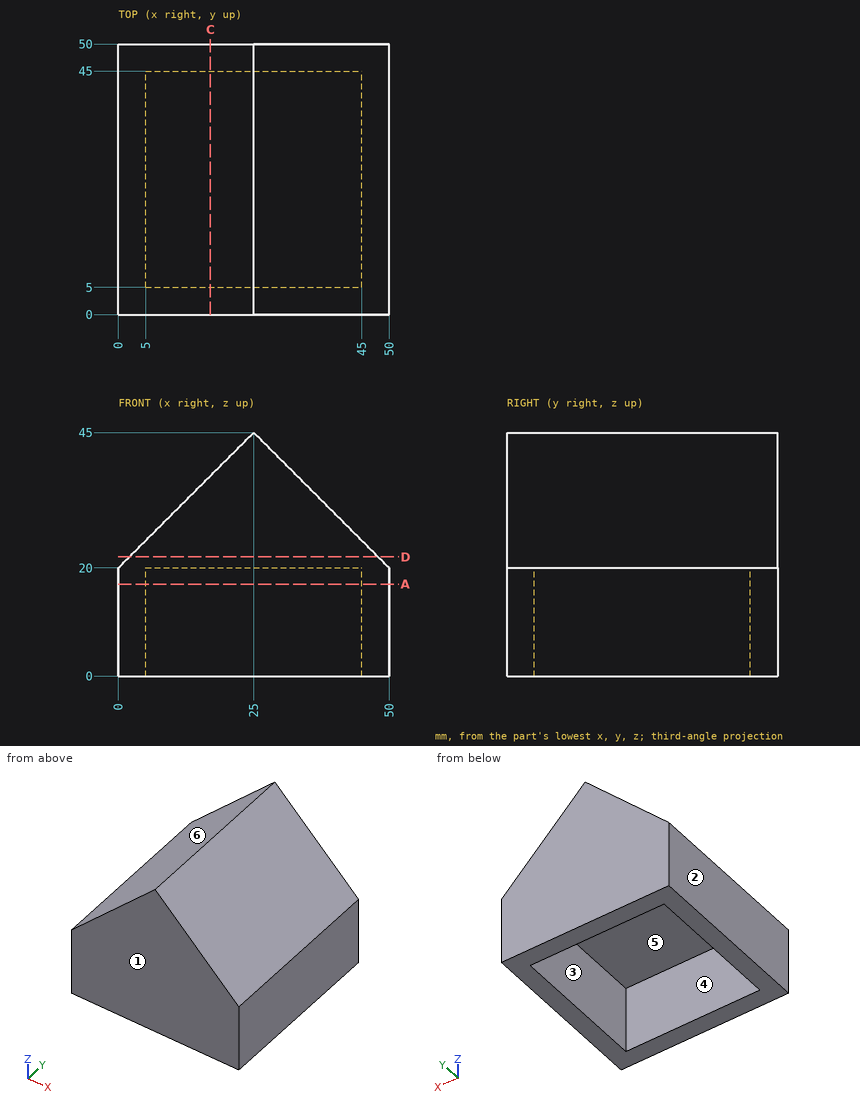
The drawing under review shows one solid part. Ordinate dimensions are in mm from its lowest x, y, z. A direction names the side the tool comes from. Coordinates: 2 decimals unless noted, no trailing zeros. Order: outer loops, then holes, each group sorted by start corner. A loop starts at its lowest first (then second) coordinate and runs counter-clockwise, first axis right, second up. Notation, with made-up numbers: (21, -5) -> (64, -5) arc R18 ccw to (64, 15) -> close; hole circle Ø5 at (10, 57.25). An arc over 180 degrees is marked (long way). Return JSON: item names as keys, results as strings.
1. For line 1 (Y direction, x = 21.5, z = 7.5); line 2 (Z direction, x = 22.5, y = 13), list the stretches that pass through material, from the lowest coordinate up. Write a range as from..to.
Answer block:
{"line 1": "0..5, 45..50", "line 2": "20..42.5"}
2. Machinability: for the marked faces 5 and 6, which of the approach directions +Z, -Z, +X, -X, +Y, -Y give a long, thin tool a straight path to every point of the face, cutting with its end or side? Answer none if there is none.
Answer block:
{"face 5": "-Z", "face 6": "+Z, -X, +Y, -Y"}
3. We need section A-A on z = 17. Write out the cut boundary in (x, y).
Answer block:
{"outline": "(0, 0) -> (50, 0) -> (50, 50) -> (0, 50) -> close; hole (5, 5) -> (45, 5) -> (45, 45) -> (5, 45) -> close"}
4. We need section D-D on z = 22. Write out the cut boundary in (x, y), and give its area (3 significant figures).
Answer block:
{"outline": "(2, 0) -> (48, 0) -> (48, 50) -> (2, 50) -> close", "area": "2,300 mm²"}
5. We need section C-C on x = 17. Write out the cut boundary in (y, z), and give its area (3 significant figures).
Answer block:
{"outline": "(0, 0) -> (5, 0) -> (5, 20) -> (45, 20) -> (45, 0) -> (50, 0) -> (50, 37) -> (0, 37) -> close", "area": "1,050 mm²"}
6. The part is to be moulded in two halves that separate along X. For the marked faces 1, 2, 3 and 4, say which applies: +X half, -X half, draft (parallel to the pull), parting line (faces both ways), or undercut.
Answer block:
{"face 1": "draft", "face 2": "-X half", "face 3": "undercut", "face 4": "undercut"}
7. For pin 1 Ø3 at (y, z) = (8.5, 26.5) entering from +X; pin 2 Ø3 at (x, z) = (31.5, 33) entering from -Y; pin 3 Ø10 at (x, y) = (18, 33.5) entering from +Z; pin 4 Ø12 at (x, y) = (32, 16.5) entering from -Z, all flat-tipped, find the tip position at first contact; note any pin that passes through.
Answer block:
{"pin 1": "x = 45", "pin 2": "y = 0", "pin 3": "z = 43", "pin 4": "z = 20"}
